Can you work these out from the drawing? Everything is in mm from the part's minimum corner. A direction names the side the tool comes from. Coordinates: 2 decimals unless noted, no trailing zeros. Loops run counter-clockwise (first coordinate to the right, second up) from the corner with the lowest first, then second, coordinate; pieces in that order, holes last.
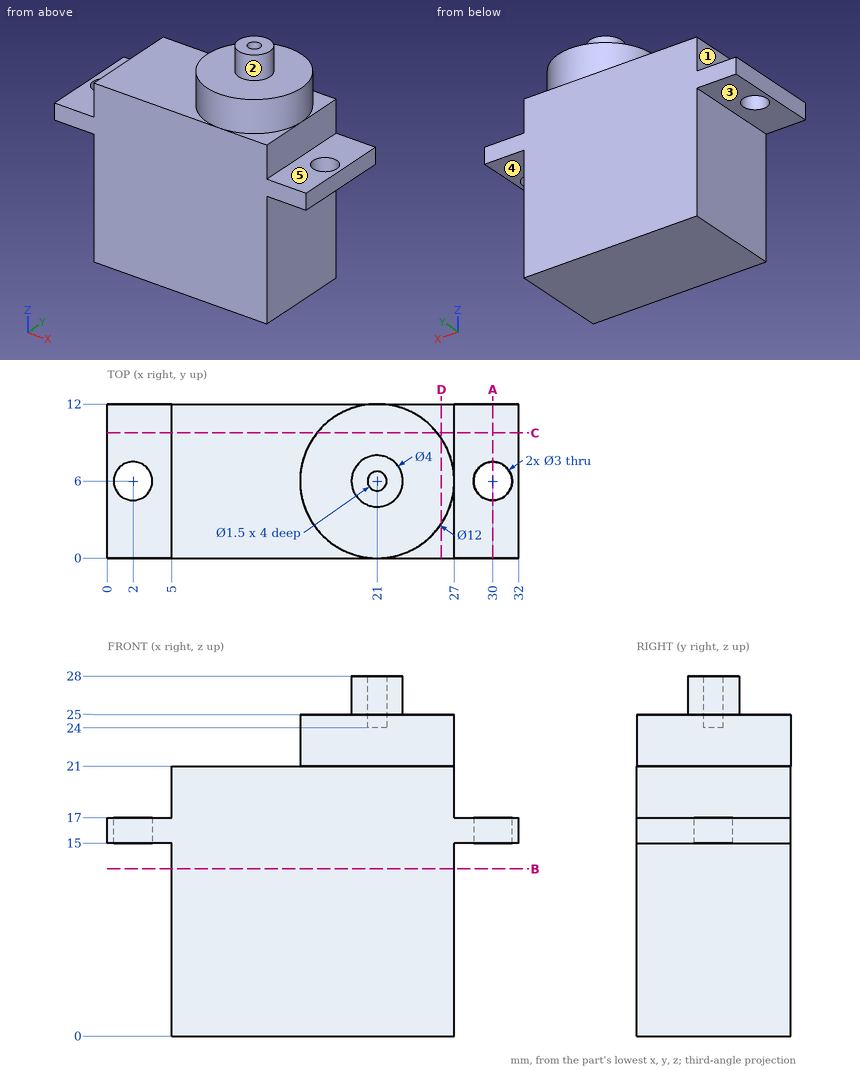
(1) I need wall thicknesses on probe 1 along Y at (x, z) = (2, 16.4); probe 2 along X at (y, z) = (1.75, 10.5); probe 3 along Z at (x, y) = (3, 4.75). Which ranges of each line are inside material? Lowest first, please.
Answers:
probe 1: y = 0 to 4.5, 7.5 to 12
probe 2: x = 5 to 27
probe 3: z = 15 to 17
(2) Imagine slicing it at A-A, the plane x = 30. Write out the boundary of the cut face in (y, z), and give its area (3 significant figures).
Answers:
outline: (0, 15) - (4.5, 15) - (4.5, 17) - (0, 17) - close; (7.5, 15) - (12, 15) - (12, 17) - (7.5, 17) - close
area: 18.0 mm2
(3) For pin 1 (2.5 mm diameter, centred on x = 30.5, y = 3, fed in from -Z); pin 2 (1.5 mm diameter, centred on x = 10.5, y = 8, fed in from -Z); pin 3 (1.8 mm diameter, centred on x = 2, y = 6, fed in from -Z); pin 4 (4 mm diameter, centred on x = 3.5, y = 4.5, fed in from +Z), each with a flat end and sliding along its axis, tell me the tip position at first contact or that it passes through.
Answers:
pin 1: stops at z = 15
pin 2: stops at z = 0
pin 3: passes through
pin 4: stops at z = 21
(4) Imagine slicing it at B-B, the plane z = 13. Write out the boundary of the cut face in (x, y).
Answers:
outline: (5, 0) - (27, 0) - (27, 12) - (5, 12) - close
(5) Imagine slicing it at D-D, the plane x = 26. Write out the boundary of the cut face in (y, z), and give its area (3 significant figures).
Answers:
outline: (0, 0) - (12, 0) - (12, 21) - (9.32, 21) - (9.32, 25) - (2.68, 25) - (2.68, 21) - (0, 21) - close
area: 279 mm2
(6) Which directions (+Z, -Z, +X, -X, +Y, -Y) give clear straight access to the entire face, cutting with the end or side of a thin tool? Please do the marked faces 1, 2, 3, 4 and 5.
Answers:
face 1: +Z, -X, +Y, -Y
face 2: +Z
face 3: -Z, -X, +Y, -Y
face 4: -Z, +X, +Y, -Y
face 5: +Z, +X, +Y, -Y
(7) Imagine slicing it at C-C, the plane y = 9.75. Write out the boundary of the cut face in (x, z).
Answers:
outline: (0, 15) - (5, 15) - (5, 0) - (27, 0) - (27, 15) - (32, 15) - (32, 17) - (27, 17) - (27, 21) - (25.68, 21) - (25.68, 25) - (16.32, 25) - (16.32, 21) - (5, 21) - (5, 17) - (0, 17) - close
